from build123d import *

# Parameters (mm, degrees)
CUT_EXTRUDE1_DEPTH      = 17
CUT_EXTRUDE1_DEPTH_BACK = 17


with BuildPart() as part:
    # Sketch1 → Revolve1 (revolve)
    with BuildSketch(Plane(origin=(0, 0, 0), x_dir=(0, 0, -1), z_dir=(1, 0, 0))):
        Polygon((-35.8, 0), (-35.8, 9.717157288), (-35.517157288, 10), (206.333333333, 10), (206.333333333, 25), (223, 25), (223, 0), align=None)
    revolve(axis=Axis((0, 0, -223), (0, 0, 1)))

    # Sketch2 → Cut-Extrude1 (cut, two sides)
    with BuildSketch(Plane(origin=(0, 0, 0), x_dir=(1, 0, 0), z_dir=(0, 1, 0))) as cut_extrude1_sk:
        Polygon((-17, -61.8), (17, -61.8), (17, -27.8), (8.5, -27.8), (8.5, -43.8), (-8.5, -43.8), (-8.5, -27.8), (-17, -27.8), align=None)
    extrude(amount=CUT_EXTRUDE1_DEPTH, mode=Mode.SUBTRACT)
    extrude(cut_extrude1_sk.sketch, amount=-CUT_EXTRUDE1_DEPTH_BACK, mode=Mode.SUBTRACT)

    # Sketch3 → Revolve2 (revolve)
    with BuildSketch(Plane(origin=(0, 0, 0), x_dir=(0, 0, -1), z_dir=(1, 0, 0))):
        with BuildLine():
            Line((-67.8, 0), (-67.8, 7.08))
            Line((-67.8, 7.08), (-66.88, 8))
            Line((-66.88, 8), (-41.28485129, 8))
            Line((-41.28485129, 8), (-38.524269872, 6.995230534))
            ThreePointArc((-38.524269872, 6.995230534), (-38.397990898, 6.961394185), (-38.267754764, 6.95))
            Line((-38.267754764, 6.95), (-36.55, 6.95))
            ThreePointArc((-36.55, 6.95), (-36.019669914, 7.169669914), (-35.8, 7.7))
            Line((-35.8, 7.7), (-35.05, 7.7))
            Line((-35.05, 7.7), (-35.05, 0))
            Line((-35.05, 0), (-67.8, 0))
        make_face()
    revolve(axis=Axis((0, 0, 35.05), (0, 0, 1)))


solid = part.part
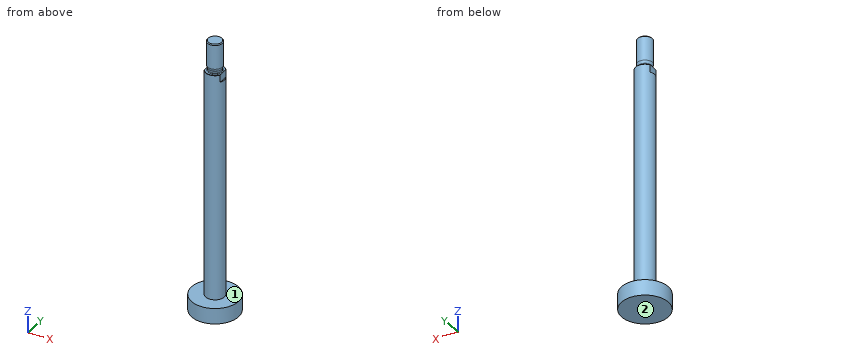
Geometry: final body of the model. Coordinates: model frame, mm. Face numbers are marked on the shaded views. A direction names the side the tool comes from. Round coordinates to 2 decimals unless told otherwise and drop trailing zeros. Loops run counter-clockwise (first coordinate to the right, second up) from the corner with the lowest first, then second, coordinate; pieces in that order, holes last.
Q1. Material intervals for L1, parallel to X at y = 2.5, z = -144.5; L2, parallel to Z at x = 21, y = 4; L3, parallel to X at y = 1, z = -154.5, sorted ascending.
Q2. Section B-B on z = -81. Return loops of the section in (x, y).
Q3. Access query for the marked faces 1 and 2. Directions: +Z, -Z, +X, -X, +Y, -Y. A direction counts if a zero-diameter tool reaches every point of the face in a straight line with its end or side. Return the directions, or none.
Q4. Section A-A on y = 0. Return loops of the section in (x, z), plus the area to 3 significant figures.
Q5. Pin query (flat end, axial travel): P1, Ø4, axis at y = 2, z = 32, coming from the +X side; P2, Ø3, axis at x = -16, y = 20, coming from the +Z side; P3, Ø0.8, axis at x = -9.5, y = 0.5, coming from the +Z side. Return the tip coordinate at first contact, or that it passes through.
Q6. Section C-C on x = -14.5. Return loops of the section in (y, z).
Q7. Section D-D on y = -21. Return loops of the section in (x, z), plus the area to 3 significant figures.
Evaluation:
1. L1: x = -9.68 to 9.68
1. L2: z = -223 to -206.33
1. L3: x = -9.95 to 9.95
2. outline: circle Ø20 at (0, 0)
3. face 1: +Z
3. face 2: -Z, +X, -X, +Y, -Y
4. outline: (-25, -223) - (25, -223) - (25, -206.33) - (10, -206.33) - (10, 27.8) - (8.5, 27.8) - (8.5, 35.8) - (7.7, 35.8) arc R0.75 cw to (6.95, 36.55) - (6.95, 38.27) arc R0.75 cw to (7, 38.52) - (8, 41.28) - (8, 66.88) - (7.08, 67.8) - (-7.08, 67.8) - (-8, 66.88) - (-8, 41.28) - (-7, 38.52) arc R0.75 cw to (-6.95, 38.27) - (-6.95, 36.55) arc R0.75 cw to (-7.7, 35.8) - (-8.5, 35.8) - (-8.5, 27.8) - (-10, 27.8) - (-10, -206.33) - (-25, -206.33) - close
4. area: 6,150 mm2
5. P1: stops at x = 8.5
5. P2: stops at z = -206.33
5. P3: stops at z = 27.8
6. outline: (-20.37, -223) - (20.37, -223) - (20.37, -206.33) - (-20.37, -206.33) - close
7. outline: (-13.56, -223) - (13.56, -223) - (13.56, -206.33) - (-13.56, -206.33) - close
7. area: 452 mm2
